from build123d import *

# Parameters (mm, degrees)
CROQUIS1_W              = 12
CROQUIS1_H              = 6
CROQUIS1_W_2            = 5
CROQUIS1_H_2            = 8
SALIENTE_EXTRUIR1_DEPTH = 2
CROQUIS2_R              = 1.25
SALIENTE_EXTRUIR2_DEPTH = 3


with BuildPart() as part:
    # Croquis1 → Saliente-Extruir1 (new body)
    with BuildSketch(Plane(origin=(0, 0, 0), x_dir=(1, 0, 0), z_dir=(0, 1, 0))):
        Polygon((0, 70), (6.7, 70), (6.7, 49), (54.7, 49), (54.7, 70), (102, 70), (102, 48), (93, 48), (93, 31), (102, 31), (102, 0), (0, 0), align=None)
        with Locations((30, 13)):
            Rectangle(CROQUIS1_W, CROQUIS1_H, mode=Mode.SUBTRACT)
        with Locations((53.5, 11)):
            Rectangle(CROQUIS1_W_2, CROQUIS1_H_2, mode=Mode.SUBTRACT)
    extrude(amount=SALIENTE_EXTRUIR1_DEPTH)

    # Croquis2 → Saliente-Extruir2 (add)
    with BuildSketch(Plane(origin=(0, 2, 0), x_dir=(1, 0, 0), z_dir=(0, 1, 0))):
        with Locations((1.9, 67.1)):
            Circle(CROQUIS2_R)
        with Locations((1.9, 36.1)):
            Circle(CROQUIS2_R)
        with Locations((76.9, 36.1)):
            Circle(CROQUIS2_R)
        with Locations((76.9, 67.1)):
            Circle(CROQUIS2_R)
    extrude(amount=SALIENTE_EXTRUIR2_DEPTH)


solid = part.part
Work out the finished part from the listing and answer in its coordinate system (mm). A direction names the side the tool comes from. Coordinates: 2 decimals unless noted, no trailing zeros. Loops run counter-clockwise (first coordinate to the right, second up) from the corner with the lowest first, then second, coordinate; pieces in that order, holes last. Notation, with made-up numbers: (20, 83.5) -> (65, 83.5) arc R8 ccw to (65, 93.5) -> close; hole circle Ø6 at (85, -2.5). An arc over 180 degrees is marked (long way). Write each question's results on one line, items separated by ' | '. Start each with the question number.
1) Find section C-C on y = 3.7. Determine the outline of the cut face in (x, z).
2) Flat-ended cylindrical pins translate along their axes: P1, Ø2, axis at x = 34.5, y = 1, coming from the -Z side; P2, Ø2, axis at x = 54.5, y = 0.5, coming from the +Z side; P3, Ø1, axis at y = 1, z = -36.5, coming from the +X side; P4, Ø1.5, axis at y = 4.5, z = -54.5, coming from the +X side. Find the tip coordinate at first contact, or state that the pin passes through.
3) For faces 5 (the flat face through (97, 1, -31)), 6 (the cylindrical face through (77.477, 3.479, -34.991)), 7 (the flat face through (54.7, 1, -59)), 8 (the flat face through (30, 1, -10)), determine the directions among +Z, -Z, +X, -X, +Y, -Y from which every point of the face is accessible in a straight line to the end or side of a thin tool.
4) Find section B-B on x = 76.9. Determine the outline of the cut face in (y, z), then the cut area to 3 significant figures.
5) Find section D-D on z = -36.1. Determine the outline of the cut face in (x, y).
6) Consider line 1 along X through (y, z) = (1.9, -49.5); line 2 along X through (y, z) = (0.45, -14.5); line 3 along Y through (x, z) = (60.5, -12). Determine where each line is inside the solid, lowest interval first.
7) Find section A-A on z = -51.5. Determine the outline of the cut face in (x, y).
8) The mould has two halves that part along Z. Classify faces 1 (the flat face through (36, 1, -13)), 2 (the flat face through (102, 1, -16)), 3 (the flat face through (30, 1, -49)), 4 (the flat face through (98, 1, -48)): pulls with the +Z half, pulls with the -Z half, needs draft (parallel to the pull), parting line crosses it, or undercut.
Response values:
1) outline: circle Ø2.5 at (1.9, -67.1); circle Ø2.5 at (1.9, -36.1); circle Ø2.5 at (76.9, -67.1); circle Ø2.5 at (76.9, -36.1)
2) P1: stops at z = -49 | P2: stops at z = 0 | P3: stops at x = 93 | P4: passes through
3) face 5: +X, +Y, -Y | face 6: +Y | face 7: -Z, +Y, -Y | face 8: +Y, -Y
4) outline: (0, -70) -> (2, -70) -> (2, -68.35) -> (5, -68.35) -> (5, -65.85) -> (2, -65.85) -> (2, -37.35) -> (5, -37.35) -> (5, -34.85) -> (2, -34.85) -> (2, 0) -> (0, 0) -> close | area: 155 mm^2
5) outline: (0, 0) -> (93, 0) -> (93, 2) -> (78.15, 2) -> (78.15, 5) -> (75.65, 5) -> (75.65, 2) -> (3.15, 2) -> (3.15, 5) -> (0.65, 5) -> (0.65, 2) -> (0, 2) -> close
6) line 1: x = 0 to 6.7, 54.7 to 102 | line 2: x = 0 to 24, 36 to 51, 56 to 102 | line 3: y = 0 to 2
7) outline: (0, 0) -> (6.7, 0) -> (6.7, 2) -> (0, 2) -> close; (54.7, 0) -> (102, 0) -> (102, 2) -> (54.7, 2) -> close
8) face 1: undercut | face 2: needs draft | face 3: pulls with the -Z half | face 4: undercut
